Verification items for the finished model (mm, model axes). A direction names the side the tool comes from. Give positions to 0.01 mm unless a question says otherwise; leave off trailing zeros. Loops run counter-clockwise (first coordinate to the right, second up) from the corner with the lowest first, then second, coordinate; pieces in that order, holes last. Notation, with made-up numbers: M -6.75,-0.75 L 9.25,-0.75 A31 ccw 9.25,36.25 Z; hole C 17,75 d6. An arc over 180 degrees is marked long. Put each result on its own line as item: value. Start each with the question number.
from build123d import *

# Parameters (mm, degrees)
SKETCH1_R           = 63.5
BOSS_EXTRUDE1_DEPTH = 10


with BuildPart() as part:
    # Sketch1 → Boss-Extrude1 (new body)
    with BuildSketch(Plane(origin=(0, 0, 0), x_dir=(1, 0, 0), z_dir=(0, 1, 0))):
        with BuildLine():
            ThreePointArc((19.89546001, -73.556853324), (0, 76.2), (-19.89546001, -73.556853324))
            Line((-19.89546001, -73.556853324), (-19.89546001, -112.983657034))
            Line((-19.89546001, -112.983657034), (-57.99546001, -112.983657034))
            Line((-57.99546001, -112.983657034), (-57.99546001, -137.056853324))
            Line((-57.99546001, -137.056853324), (57.99546001, -137.056853324))
            Line((57.99546001, -137.056853324), (57.99546001, -112.983657034))
            Line((57.99546001, -112.983657034), (19.89546001, -112.983657034))
            Line((19.89546001, -112.983657034), (19.89546001, -73.556853324))
        make_face()
        Circle(SKETCH1_R, mode=Mode.SUBTRACT)
    extrude(amount=BOSS_EXTRUDE1_DEPTH)


solid = part.part
Q1. Cross-section at D-D, the plane x = -26. Record the boundary of the cut face in (y, z), then the cut area to 3 significant figures.
Q2. Set-up check for faces 5 (the face through (-19.895, 5, 93)), 6 (the face through (-57.995, 5, 125)), 7 (the face through (57.995, 5, 125)): record each of +Z, -Z, +X, -X, +Y, -Y from which the full face is reachable in a straight line by a thin tool's end or side.
Q3. Cross-section at B-B, the plane z = 0. Record the boundary of the cut face in (x, y), then the cut area to 3 significant figures.
Q4. Release check for a two-part mould opening along Z. For faces 1 (the face through (39, 5, 112.984)), 2 (the face through (-17, 10, 62)), 3 (the face through (-1, 5, 137.057)), 4 (the face through (3.07, 4.93, -76.14)) record: pulls with the +Z half, pulls with the -Z half, needs draft (parallel to the pull), parting line crosses it, or undercut.
Q5. Scan lines: L1, parallel to Z at x = -28.5, y = 8; L2, parallel to X at y = 7.75, z = 0; L3, parallel to Z at x = -38, y = 2.25. Record each from-to range of solid material in increasing order.
Q6. Cross-section at A-A, the plane x = 0. Record the boundary of the cut face in (y, z), then the cut area to 3 significant figures.
Q7. Cross-section at C-C, the plane y = 6.5. Record the boundary of the cut face in (x, z).
Q8. Go/stop test with flat-tipped pins: pin 1 (1 mm diameter, centred on y = 8.5, z = 50.5, fed in from -X); pin 2 (4 mm diameter, centred on x = -53, y = 3, fed in from -Z); pin 3 (5 mm diameter, centred on y = 4.5, z = 88, fed in from +X). Record where each tip stops, or that it passes through.
Ans:
1. outline: M 0,-71.63 L 10,-71.63 L 10,-57.93 L 0,-57.93 Z; M 0,57.93 L 10,57.93 L 10,71.63 L 0,71.63 Z; M 0,112.98 L 10,112.98 L 10,137.06 L 0,137.06 Z
1. area: 515 mm^2
2. face 5: -X, +Y, -Y
2. face 6: +Z, -X, +Y, -Y
2. face 7: +Z, +X, +Y, -Y
3. outline: M -76.2,0 L -63.5,0 L -63.5,10 L -76.2,10 Z; M 63.5,0 L 76.2,0 L 76.2,10 L 63.5,10 Z
3. area: 254 mm^2
4. face 1: undercut
4. face 2: needs draft
4. face 3: pulls with the +Z half
4. face 4: undercut
5. L1: z = -70.67 to -56.75, 56.75 to 70.67, 112.98 to 137.06
5. L2: x = -76.2 to -63.5, 63.5 to 76.2
5. L3: z = -66.05 to -50.87, 50.87 to 66.05, 112.98 to 137.06
6. outline: M 0,-76.2 L 10,-76.2 L 10,-63.5 L 0,-63.5 Z; M 0,63.5 L 10,63.5 L 10,137.06 L 0,137.06 Z
6. area: 863 mm^2
7. outline: M -58,112.98 L -19.9,112.98 L -19.9,73.56 A76.2 ccw long 19.9,73.56 L 19.9,112.98 L 58,112.98 L 58,137.06 L -58,137.06 Z; hole C 0,0 d127
8. pin 1: stops at x = -57.5
8. pin 2: stops at z = -56.62
8. pin 3: stops at x = 19.9
